Design review of the part built by this model. Coordinates are the model's own, in mm. A direction names the side the tool comes from. Round coordinates to 2 decimals unless told otherwise and drop trailing zeros. Order: outer loops, then holes, each group sorted by start corner. A loop starts at its lowest first (then second) coordinate and runs counter-clockwise, first axis right, second up. Notation, with made-up numbers: (21, 59.25) - (28, 59.25) arc R27 cw to (28, 91.25) - close; hole circle Ø2 at (66.25, -18). An arc over 180 degrees is marked (long way). Use CSV: the item, a comma, the result in double quotes.
Solid Edge part; units mm, degrees
sketch "Sketch1" plane through (0, 0, 0) normal (0, 0, 1) x (1, 0, 0)
  circle A0 centre (0, 0) radius 7.1374
extrude "Protrusion1" add sketch "Sketch1" along normal blind 6.35
sketch "Sketch2" plane through (0, 0, 0) normal (0, 0, -1) x (0, 1, 0)
  circle A0 centre (0, 0) radius 4.7625
extrude "Protrusion2" add sketch "Sketch2" along normal blind 15.875
sketch "Sketch3" plane through (0, 0, -15.875) normal (0, 0, -1) x (0, 1, 0)
  circle A0 centre (0, 0) radius 3.9688
extrude "Protrusion3" add sketch "Sketch3" along normal blind 12.7
sketch "Sketch4" plane through (0, 0, 6.35) normal (0, 0, 1) x (0, 1, 0)
  line L0 (-2.3876, 1.3131) -> (0, 2.8792)
  line L1 (-2.3876, -1.5424) -> (-2.3876, 1.3131)
  line L2 (-2.3876, -1.5424) -> (0, -2.8792)
  line L3 (2.3876, -1.5424) -> (0, -2.8792)
  line L4 (2.3876, -1.5424) -> (2.3876, 1.3131)
  line L5 (2.3876, 1.3131) -> (0, 2.8792)
extrude "Cutout1" cut sketch "Sketch4" against normal blind 3.175
chamfer "Chamfer1" distance 0.7874 angle 45 1 edges at (0, -3.9688, -28.575)
properties part number "163434"
1) The part is to be moulded in two halves that separate along Y. For faces 1 (the face through (1.52, 3.666, -21.748)), 2 (the face through (0, 0, 3.175)), 3 (the face through (1, -5, 0)), say which applies: +Y half, -Y half, draft (parallel to the pull), parting line (faces both ways), or undercut.
Data:
face 1,"parting line"
face 2,"undercut"
face 3,"draft"
2) To check wall thickness, follow L1, parallel to X at y = 0, z = -4; L2, parallel to Z at x = -1, y = -0.25 (3 decimals); L3, parallel to Z at x = 4, y = -4. State the ranges of each line that lie inside material, in increasing order. Write a range as from..to.
Data:
L1,"x = -4.76..4.76"
L2,"z = -28.575..3.175"
L3,"z = 0..6.35"
3) We need section A-A (z = -2.5). Give the boundary of the cut face in (x, y) (1 decimal).
Data:
outline,"circle Ø9.5 at (0, 0)"
4) We need section C-C (y = -5.5). Give the boundary of the cut face in (x, z).
Data:
outline,"(-4.55, 0) - (4.55, 0) - (4.55, 6.35) - (-4.55, 6.35) - close"
5) We need section D-D (z = -18). Give the boundary of the cut face in (x, y).
Data:
outline,"circle Ø7.94 at (0, 0)"
6) We need section B-B (x = 5.75). Give the boundary of the cut face in (y, z), then the cut area to 3 significant figures.
Data:
outline,"(-4.23, 0) - (4.23, 0) - (4.23, 6.35) - (-4.23, 6.35) - close"
area,"53.7 mm2"
7) For faces 4 (the face through (2, 4, -15.875)), 5 (the face through (2.2, 1.21, 4.78)), 6 (the face through (0, 0, -28.575)), list the 3-axis set-ups (+Z, -Z, +X, -X, +Y, -Y) from which the entire face can be reached by the end or side of a thin tool; tool diameter is ignored.
Data:
face 4,"-Z"
face 5,"+Z"
face 6,"-Z, +X, -X, +Y, -Y"
8) Insertion check: pin 1 Ø3 at (x, z) = (0.5, 4.5) entering from +Y; pin 2 Ø2 at (x, z) = (0.5, -22.5) entering from +Y; pin 3 Ø1.4 at (x, z) = (1, 4.5) entering from -Y; pin 4 Ø1 at (x, z) = (0, -15.5) entering from +Y. Each pin has a flat end and moves straight along its axis. Give the tip position at first contact, or say it passes through.
Data:
pin 1,"stops at y = 7.14"
pin 2,"stops at y = 3.97"
pin 3,"stops at y = -7.13"
pin 4,"stops at y = 4.76"
